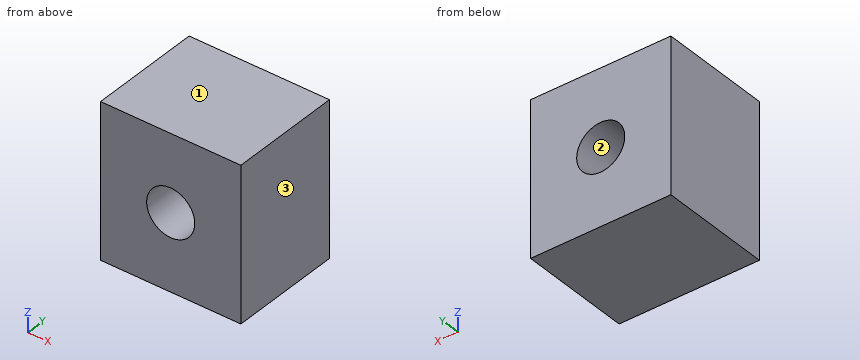
```python
from build123d import *

# Parameters (mm, degrees)
F0_W     = 31.5161347389
F0_H     = 34.4433300197
F0_R     = 5.3996855878
F1_DEPTH = 25.4


# Not quite as in the source:
# - the program builds the solid bodies; features that only make, move or delete a surface that nothing else refers to are left out


with BuildPart() as f1:
    # F0 (on Front) → F1 (new body)
    with BuildSketch(Plane.XZ):
        Rectangle(F0_W, F0_H)
        Circle(F0_R, mode=Mode.SUBTRACT)
    extrude(amount=F1_DEPTH)


solid = f1.part
```
Here's how the part is built. I have some questions about the finished solid (model axes, mm). Face numbers are marked on the shaded views. Coordinates: 2 decimals unless noted, no trailing zeros. Order: outer loops, then holes, each group sorted by start corner. A loop starts at its lowest first (then second) coordinate and runs counter-clockwise, first axis right, second up.
1) I need wall thicknesses on line 1 (Z direction, x = 0, y = -8.75); line 2 (X direction, y = -16.75, z = 3.5); line 3 (Z direction, x = 1, y = -6). Which ranges of each line are inside material? Lowest first, please.
2) Imagine slicing it at A-A on x = 0. List the corners of the cut face in (y, z) for me.
3) Imagine slicing it at B-B on z = 0. List the corners of the cut face in (x, y) for me.
4) We'd pull the mould along Z, two halves only. Please class the marked faces 1, 2 and 3: +Z half, -Z half, draft (parallel to the pull), parting line (faces both ways), or undercut.
5) Imagine slicing it at C-C on y = -14. List the corners of the cut face in (x, z) for me, and give its area (3 significant figures).
Response values:
1. line 1: z = -17.22 to -5.4, 5.4 to 17.22
1. line 2: x = -15.76 to -4.11, 4.11 to 15.76
1. line 3: z = -17.22 to -5.31, 5.31 to 17.22
2. outline: (-25.4, -17.22) - (0, -17.22) - (0, -5.4) - (-25.4, -5.4) - close; (-25.4, 5.4) - (0, 5.4) - (0, 17.22) - (-25.4, 17.22) - close
3. outline: (-15.76, -25.4) - (-5.4, -25.4) - (-5.4, 0) - (-15.76, 0) - close; (5.4, -25.4) - (15.76, -25.4) - (15.76, 0) - (5.4, 0) - close
4. face 1: +Z half
4. face 2: undercut
4. face 3: draft
5. outline: (-15.76, -17.22) - (15.76, -17.22) - (15.76, 17.22) - (-15.76, 17.22) - close; hole circle Ø10.8 at (0, 0)
5. area: 994 mm2
